Autodesk Inventor part; units mm, degrees
ref_plane "YZ Plane" through (0, 0, 0) normal (1, 0, 0) x (0, 1, 0)
ref_plane "XZ Plane" through (0, 0, 0) normal (0, 1, 0) x (-1, 0, 0)
ref_plane "XY Plane" through (0, 0, 0) normal (0, 0, 1) x (1, 0, 0)
sketch "Sketch1" plane through (0, 0, 0) normal (0, 0, 1) x (1, 0, 0)
  line L0 (0, 0) -> (0, 88.9)
  line L1 (0, 88.9) -> (467.8791, 0)
  line L2 (467.8791, 0) -> (0, 0)
  dimension "d0" = 88.9
  dimension "d4" = 476.25
  dimension "d5" = 90
extrude "Extrusion1" add sketch "Sketch1" along normal blind 3.175
sketch "Sketch2" plane through (0, 88.9, 0) normal (0.1866667, 0.9824233, 0) x (0.9824233, -0.1866667, 0)
  line L0 (0, 0) -> (476.25, 0)
  line L1 (0, 0) -> (0, -3.175)
  line L2 (476.25, -3.175) -> (0, -3.175)
  line L3 (476.25, 0) -> (476.25, -3.175)
  line L4 (0, -3.175) -> (0, -330.2)
  line L5 (0, -330.2) -> (476.25, -330.2)
  line L6 (476.25, -330.2) -> (476.25, -3.175)
  point P0 (16.594667, 0)
  dimension "d6" = 330.2
extrude "Extrusion2" add sketch "Sketch2" along normal blind 3.175
sketch "Sketch3" plane through (0, 0, 0) normal (-1, 0, 0) x (0, 0, 1)
  line L0 (0, 0) -> (0, 88.9)
  line L1 (0, 0) -> (3.175, 0)
  line L2 (3.175, 88.9) -> (3.175, 0)
  line L3 (0, 88.9) -> (3.175, 88.9)
  line L4 (0, 88.9) -> (0, 92.075)
  line L5 (0, 92.075) -> (330.2, 92.075)
  line L6 (330.2, 92.075) -> (330.2, 0)
  line L7 (330.2, 0) -> (330.2, -101.6)
  line L8 (330.2, -101.6) -> (0, -101.6)
  line L9 (0, -101.6) -> (0, 0)
  dimension "d9" = 3.175
  dimension "d10" = 330.2
  dimension "d11" = 101.6
extrude "Extrusion3" add sketch "Sketch3" along normal blind 3.175
sketch "Sketch4" plane through (0, 0, 0) normal (0, 0, -1) x (-1, 0, 0)
  line L0 (0, 88.9) -> (-0.592667, 92.019194)
  line L1 (0, 92.075) -> (0, 88.9)
  line L2 (-0.592667, 92.019194) -> (0, 92.075)
extrude "Extrusion4" add sketch "Sketch4" against normal blind 330.2
sketch "Sketch5" plane through (0, -101.6, 330.2) normal (0, 0, 1) x (1, 0, 0)
  line L0 (0, 190.5) -> (467.8791, 101.6)
  line L1 (467.8791, 101.6) -> (468.471767, 104.719194)
  line L2 (0.592667, 193.619194) -> (468.471767, 104.719194)
  line L3 (0.592667, 193.619194) -> (0, 193.675)
  line L4 (0, 193.675) -> (-3.175, 193.675)
  line L5 (-3.175, 0) -> (-3.175, 193.675)
  line L6 (0, 0) -> (-3.175, 0)
  line L7 (0, 0) -> (0, 190.5)
  line L8 (468.471767, 104.719194) -> (468.471767, 0)
  line L9 (468.471767, 0) -> (0, 0)
  point P0 (0, 101.6)
extrude "Extrusion5" add sketch "Sketch5" along normal blind 3.175
sketch "Sketch6" plane through (0, -101.6, 330.2) normal (0, 0, -1) x (-1, 0, 0)
  line L0 (-467.8791, 101.6) -> (-468.471767, 104.719194)
  line L1 (-468.471767, 0) -> (-468.471767, 104.719194)
  line L2 (-467.8791, 101.6) -> (-468.471767, 101.6)
  point P0 (0, 101.6)
extrude "Extrusion6" add sketch "Sketch6" along normal blind 330.2
sketch "Sketch7" plane through (468.471767, -101.6, 330.2) normal (1, 0, 0) x (0, 0, -1)
  line L0 (0, 0) -> (0, 101.6)
  line L1 (0, 101.6) -> (330.2, 101.6)
  line L2 (330.2, 104.719194) -> (330.2, 101.6)
  line L3 (-3.175, 104.719194) -> (330.2, 104.719194)
  line L4 (-3.175, 0) -> (-3.175, 104.719194)
  line L5 (0, 0) -> (-3.175, 0)
  line L6 (0, 0) -> (330.2, 0)
  line L7 (330.2, 0) -> (330.2, 101.6)
extrude "Extrusion7" add sketch "Sketch7" along normal blind 3.175
sketch "Sketch8" plane through (0, -101.6, 0) normal (0, -1, 0) x (1, 0, 0)
  line L0 (0, 0) -> (0, 330.2)
  line L1 (471.646767, 333.375) -> (471.646767, 0)
  line L2 (-3.175, 333.375) -> (471.646767, 333.375)
  line L3 (-3.175, 0) -> (-3.175, 333.375)
  line L4 (0, 0) -> (-3.175, 0)
  line L5 (0, 0) -> (471.646767, 0)
extrude "Extrusion8" add sketch "Sketch8" along normal blind 3.175
sketch "Sketch9" plane through (0, 88.9, 0) normal (-0.1866667, -0.9824233, 0) x (0.9824233, -0.1866667, 0)
  line L0 (0, 330.2) -> (476.25, 330.2)
  line L1 (0, 3.175) -> (0, 330.2)
  arc A0 (0, 184.15) -> (146.05, 330.2) centre (146.05, 184.15) ccw
  point P0 (16.594667, 0)
  dimension "d24" = 292.1
extrude "Extrusion9" cut sketch "Sketch9" against normal blind 3.175
sketch "Sketch10" plane through (471.646767, -101.6, 330.2) normal (1, 0, 0) x (0, 0, -1)
  line L0 (330.2, 104.719194) -> (-3.175, 104.719194)
  line L1 (-3.175, 104.719194) -> (-3.175, -3.175)
  line L2 (330.2, -3.175) -> (-3.175, -3.175)
  line L3 (123.825, 53.919194) -> (123.825, 206.319194)
  line L4 (123.825, 206.319194) -> (-79.375, 206.319194)
  line L5 (123.825, 53.919194) -> (-3.175, 53.919194)
  line L6 (-3.175, 53.919194) -> (-3.175, 104.719194)
  line L7 (-3.175, 104.719194) -> (-3.175, 104.719194)
  line L8 (-3.175, 104.719194) -> (-79.375, 206.319194)
  point P0 (330.2, 101.6)
  dimension "d30" = 152.4
  dimension "d31" = 203.2
  dimension "d32" = 127
  dimension "d33" = 50.8
  dimension "d34" = 0
  dimension "d35" = 0
  dimension "d47" = 0
extrude "Extrusion10" add sketch "Sketch10" along normal blind 3.175
sketch "Sketch11" plane through (-3.175, 0, 0) normal (-1, 0, 0) x (0, 0, 1)
  line L0 (333.375, 92.075) -> (333.375, -104.775)
  line L1 (0, 92.075) -> (333.375, 92.075)
  line L2 (311.15, 206.375) -> (31.75, 206.375)
  line L3 (311.15, 206.375) -> (311.15, 41.275)
  line L4 (311.15, 41.275) -> (101.6, 41.275)
  line L5 (101.6, 41.275) -> (101.6, 92.075)
  line L6 (101.6, 92.075) -> (31.75, 206.375)
  point P0 (0, 0)
  dimension "d39" = 279.4
  dimension "d40" = 165.1
  dimension "d41" = 209.55
  dimension "d42" = 50.8
  dimension "d43" = 0
  dimension "d44" = 22.225
extrude "Extrusion11" add sketch "Sketch11" along normal blind 3.175
properties part number "Hopper" material "Glass"
Part model, mm, in its own coordinate system. A direction names the side the tool comes from. Coordinates: 2 decimals unless noted, no trailing zeros. Loops run counter-clockwise (first coordinate to the right, second up) from the corner with the lowest first, then second, coordinate; pieces in that order, holes last. Notation, with made-up numbers: M 48.25,45 L 84.25,45 A25 ccw 84.25,68 Z; hole C 55,-15 d5. An arc over 180 degrees is marked long. Use a Markdown table: item, result. Add a question column.
Q1. Pin check, flat tips, straight feed: P1, Ø3.5, axis at x = 473, y = 22, coming from the -Z side (3 decimals); P2, Ø4, axis at y = -13.5, z = 148, coming from the -X side (3 decimals); P3, Ø1, axis at x = 241, y = -11.5, coming from the -Z side; P4, Ø3, axis at x = 89, y = 20, coming from the -Z side. Stop position of each tip, or through.
Q2. Cut at C-C (z = 116). Write the cut outline in (x, y) (3 decimals).
Q3. Cut at D-D (x = 293.5). Write the cut outline in (y, z) (3 decimals).
Q4. Which spindle directions (+Z, -Z, +X, -X, +Y, -Y) get a long thin tool onto all of the face, cutting with end or side? Do faces 5 (the flat face through (231, -25, 330.2)), 6 (the flat face through (471.647, 55, 287)), 7 (the flat face through (473.212, 53.208, 370.942)), 8 (the flat face through (231, -104.775, 169)), 9 (the flat face through (231, -101.6, 167)). Say none if no direction does.
Q5. Cut at B-B (y = -14). Write the cut outline in (x, z) (3 decimals).
Q6. Probe L1, parallel to X at y = -46.5, z = 303 (3 decimals); L2, parallel to X at y = -69.5, z = 257 (3 decimals); L3, parallel to Y at x = 154, z = 158.5 (3 decimals). List the from-to ranges inside material, lowest first.
Q7. Mould opens along X. For faces 1 (the flat face through (-6.35, 125, 201)), 2 (the flat face through (474.822, 30, 287)), 3 (the flat face through (468.472, -50, 167)), 4 (the flat face through (334.638, 25.317, 128.062)) say: +X half, -X half, draft (parallel to the pull), parting line (faces both ways), or undercut.
Worked out:
| question | item | result |
|---|---|---|
| 1 | P1 | stops at z = 206.375 |
| 1 | P2 | stops at x = -3.175 |
| 1 | P3 | stops at z = 330.2 |
| 1 | P4 | stops at z = 0 |
| 2 | outline | M -6.35,41.275 L -3.175,41.275 L -3.175,-104.775 L 471.647,-104.775 L 471.647,3.119 L 468.472,3.119 L 270.98,40.644 L 270.387,37.525 L 467.879,0 L 468.472,0 L 468.472,-101.6 L 0,-101.6 L 0,88.9 L 16.578,85.75 L 17.171,88.869 L 0.593,92.019 L 0,92.075 L -3.175,92.075 L -3.175,206.375 L -6.35,206.375 Z |
| 3 | outline | M -104.775,0 L -101.6,0 L -101.6,330.2 L 33.133,330.2 L 33.133,3.175 L 0,3.175 L 0,0 L 36.365,0 L 36.365,333.375 L -104.775,333.375 Z |
| 4 | face 5 | none |
| 4 | face 6 | +Z, -Z, +Y |
| 4 | face 7 | +Z, +X, -X, -Y |
| 4 | face 8 | +Z, -Z, +X, -X, -Y |
| 4 | face 9 | -Z |
| 5 | outline | M -3.175,0 L 0,0 L 0,330.2 L 468.472,330.2 L 468.472,0 L 471.647,0 L 471.647,206.375 L 474.822,206.375 L 474.822,333.375 L -3.175,333.375 Z |
| 6 | L1 | x = -3.175 to 0, 468.472 to 474.822 |
| 6 | L2 | x = -3.175 to 0, 468.472 to 471.647 |
| 6 | L3 | y = -104.775 to -101.6 |
| 7 | face 1 | -X half |
| 7 | face 2 | +X half |
| 7 | face 3 | undercut |
| 7 | face 4 | undercut |
